Verification items for the finished model (mm, model axes). Face numbers are marked on the shaded views. A direction names the side the tool comes from. Give positions to 0.01 mm unless a question says otherwise; leave off trailing zeros. Write each loop counter-clockwise with the first axis right and the second up, starting at its lowest first coordinate (ties: lowest second). Pieces come first, ordered by that corner, then holes. Notation, with made-up numbers: M 13,3.5 L 69,3.5 A14 cw 69,24.5 Z; hole C 55.5,21.5 d6. An arc over 180 degrees is marked long. Answer as a JSON object with one key per item and string values.
```python
from build123d import *

# Parameters (mm, degrees)
SKETCH1_R           = 11.25
SKETCH1_R_2         = 1.6
BOSS_EXTRUDE1_DEPTH = 5
SKETCH4_R           = 2.8
CUT_EXTRUDE1_DEPTH  = 2.5
BOSS_EXTRUDE2_START = 11
SKETCH2_R           = 2.8
BOSS_EXTRUDE2_DEPTH = 11
BOSS_EXTRUDE3_DEPTH = 3
CHAMFER2_SIZE       = 1
CUT_EXTRUDE2_REACH  = 42.599
SKETCH5_R           = 2.1
SKETCH6_R           = 3.5
CUT_EXTRUDE3_DEPTH  = 7
CHAMFER3_SIZE       = 0.75


with BuildPart() as part:
    # Sketch1 → Boss-Extrude1 (new body)
    with BuildSketch(Plane(origin=(0, 0, 0), x_dir=(1, 0, 0), z_dir=(0, 1, 0))):
        Polygon((-20, 20.75), (-15, 20.75), (-14, 21.75), (-6, 21.75), (-5, 20.75), (5, 20.75), (6, 21.75), (14, 21.75), (15, 20.75), (20, 20.75), (20, -20.75), (-20, -20.75), align=None)
        with Locations(Location((0, 0, 0), (0, 0, 270))):
            Circle(SKETCH1_R, mode=Mode.SUBTRACT)
        with Locations(Location((15.5, 15.5, 0), (0, 0, 270))):
            Circle(SKETCH1_R_2, mode=Mode.SUBTRACT)
        with Locations(Location((-15.5, 15.5, 0), (0, 0, 270))):
            Circle(SKETCH1_R_2, mode=Mode.SUBTRACT)
        with Locations(Location((-15.5, -15.5, 0), (0, 0, 270))):
            Circle(SKETCH1_R_2, mode=Mode.SUBTRACT)
        with Locations(Location((15.5, -15.5, 0), (0, 0, 270))):
            Circle(SKETCH1_R_2, mode=Mode.SUBTRACT)
    extrude(amount=BOSS_EXTRUDE1_DEPTH)

    # Sketch4 → Cut-Extrude1 (cut)
    with BuildSketch(Plane(origin=(0, 5, 0), x_dir=(1, 0, 0), z_dir=(0, 1, 0))):
        with Locations(Location((-15.5, -15.5, 0), (0, 0, 270))):
            Circle(SKETCH4_R)
        with Locations(Location((15.5, 15.5, 0), (0, 0, 270))):
            Circle(SKETCH4_R)
        with Locations(Location((-15.5, 15.5, 0), (0, 0, 270))):
            Circle(SKETCH4_R)
        with Locations(Location((15.5, -15.5, 0), (0, 0, 270))):
            Circle(SKETCH4_R)
    extrude(amount=-CUT_EXTRUDE1_DEPTH, mode=Mode.SUBTRACT)

    # Sketch2 → Boss-Extrude2 (add)
    with BuildSketch(Plane(origin=(0, 5, 0), x_dir=(1, 0, 0), z_dir=(0, 1, 0)).offset(BOSS_EXTRUDE2_START)):
        with BuildLine():
            Line((-20, 10.75), (-8.968695557, 10.75))
            ThreePointArc((-8.968695557, 10.75), (0, 14), (8.968695557, 10.75))
            Line((8.968695557, 10.75), (20, 10.75))
            Line((20, 10.75), (20, 20.75))
            Line((20, 20.75), (15, 20.75))
            Line((15, 20.75), (14, 21.75))
            Line((14, 21.75), (6, 21.75))
            Line((6, 21.75), (5, 20.75))
            Line((5, 20.75), (-5, 20.75))
            Line((-5, 20.75), (-6, 21.75))
            Line((-6, 21.75), (-14, 21.75))
            Line((-14, 21.75), (-15, 20.75))
            Line((-15, 20.75), (-20, 20.75))
            Line((-20, 20.75), (-20, 10.75))
        make_face()
        with Locations((-15.5, 15.5)):
            Circle(SKETCH2_R, mode=Mode.SUBTRACT)
        with Locations((15.5, 15.5)):
            Circle(SKETCH2_R, mode=Mode.SUBTRACT)
    extrude(amount=-BOSS_EXTRUDE2_DEPTH)

    # Sketch3 → Boss-Extrude3 (add)
    with BuildSketch(Plane(origin=(20, 0, 0), x_dir=(0, 0, -1), z_dir=(1, 0, 0))):
        Polygon((10.75, 16), (-8.302558883, 5), (10.75, 5), align=None)
    boss_extrude3 = extrude(amount=-BOSS_EXTRUDE3_DEPTH)

    # Mirror1: Boss-Extrude3 across plane
    add(boss_extrude3.mirror(Plane(origin=(0, 0, 0), x_dir=(0, 0, 1), z_dir=(1, 0, 0))))

    # Chamfer2
    chamfer2_edges = [part.edges().sort_by_distance(p)[0] for p in [
        (12.984347779, 5, -10.75),
        (17, 5, -1.223720558),
        (-17, 5, -1.223720558),
        (0, 5, -14),
        (-12.984347779, 5, -10.75),
    ]]
    chamfer(chamfer2_edges, length=CHAMFER2_SIZE)

    # Sketch5 → Cut-Extrude2 (cut, up to next)
    with BuildSketch(Plane.XY.offset(-10.75), mode=Mode.PRIVATE) as cut_extrude2_sk1:
        with Locations((-10, 11)):
            Circle(SKETCH5_R)
    cut_extrude2_tool1 = extrude(cut_extrude2_sk1.sketch, amount=-CUT_EXTRUDE2_REACH, mode=Mode.PRIVATE) & part.part
    # Sketch5 → Cut-Extrude2 (cut, up to next)
    with BuildSketch(Plane.XY.offset(-10.75), mode=Mode.PRIVATE) as cut_extrude2_sk2:
        with Locations((10, 11)):
            Circle(SKETCH5_R)
    cut_extrude2_tool2 = extrude(cut_extrude2_sk2.sketch, amount=-CUT_EXTRUDE2_REACH, mode=Mode.PRIVATE) & part.part
    add(cut_extrude2_tool1.solids().sort_by_distance((-10, 11, -10.75))[0], mode=Mode.SUBTRACT)
    add(cut_extrude2_tool2.solids().sort_by_distance((10, 11, -10.75))[0], mode=Mode.SUBTRACT)

    # Sketch6 → Cut-Extrude3 (cut)
    with BuildSketch(Plane.XY.offset(-10.75)):
        with Locations((-10, 11)):
            Circle(SKETCH6_R)
        with Locations((10, 11)):
            Circle(SKETCH6_R)
    extrude(amount=-CUT_EXTRUDE3_DEPTH, mode=Mode.SUBTRACT)

    # Chamfer3
    chamfer3_edges = [part.edges().sort_by_distance(p)[0] for p in [
        (-17.5, 0, -20.75),
        (-14.5, 0, -21.25),
        (20, 5, 14.526279442),
        (-10, 0, -21.75),
        (20, 10.5, -1.223720558),
        (-5.5, 0, -21.25),
        (0, 0, -20.75),
        (-20, 5, 14.526279442),
        (-20, 10.5, -1.223720558),
        (5.5, 0, -21.25),
        (10, 0, -21.75),
        (14.5, 0, -21.25),
        (17.5, 0, -20.75),
        (20, 0, 0),
        (0, 0, 20.75),
        (-20, 0, 0),
        (20, 2.5, 20.75),
        (-20, 2.5, 20.75),
        (0, 0, -11.25),
        (15.5, 0, -17.1),
        (-15.5, 0, -17.1),
        (-15.5, 0, 13.9),
        (15.5, 0, 13.9),
        (0, 5, 20.75),
        (0, 16, -14),
        (20, 16, -15.75),
        (17.5, 16, -20.75),
        (14.5, 16, -21.25),
        (10, 16, -21.75),
        (5.5, 16, -21.25),
        (0, 16, -20.75),
        (-5.5, 16, -21.25),
        (-10, 16, -21.75),
        (-14.5, 16, -21.25),
        (-17.5, 16, -20.75),
        (-20, 16, -15.75),
    ]]
    chamfer(chamfer3_edges, length=CHAMFER3_SIZE)


solid = part.part
```
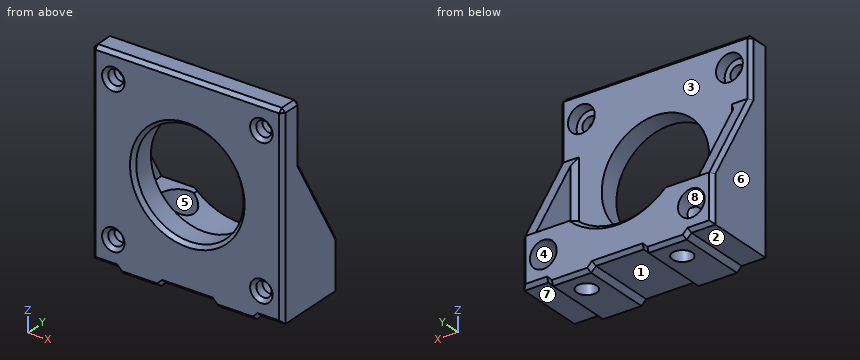
1) Access from +Z, -Z, +X, -X, +Y, -Y to the whole of each face (thin tool, end or side, straight path). Record for the marked faces 1, 2, 3, 4 and 5.
Completed:
{"face 1": "-Z, +Y, -Y", "face 2": "-Z, -X, +Y, -Y", "face 3": "+Z, +Y", "face 4": "+Y", "face 5": "+Z"}
2) Go/stop test with flat-tipped pins: pin 1 (1.5 mm diameter, centred on x = -18, y = 6, fed in from -Z); pin 2 (7.5 mm diameter, centred on x = -15.5, z = 15.5, fed in from +Y); pin 3 (2.5 mm diameter, centred on x = -11.5, y = 8.5, fed in from +Z). Record where each tip stops, or that it passes through.
Completed:
{"pin 1": "stops at z = -20.75", "pin 2": "stops at y = 5", "pin 3": "stops at z = -10.75"}
3) Section check B-B on y = 1.5. Record the boundary of the cut face in (x, z).
Completed:
{"outline": "M -20,-20.75 L -15,-20.75 L -14,-21.75 L -6,-21.75 L -5,-20.75 L 5,-20.75 L 6,-21.75 L 14,-21.75 L 15,-20.75 L 20,-20.75 L 20,20 L 19.25,20.75 L -19.25,20.75 L -20,20 Z; hole C -15.5,-15.5 d3.2; hole C -15.5,15.5 d3.2; hole C 0,0 d22.5; hole C 15.5,-15.5 d3.2; hole C 15.5,15.5 d3.2"}
4) Release check for a two-part mould opening along X. For the marked faces 6, 7 and 8 record: pulls with the +X half, pulls with the -X half, needs draft (parallel to the pull), parting line crosses it, or undercut.
Completed:
{"face 6": "pulls with the -X half", "face 7": "needs draft", "face 8": "undercut"}
5) Thickness scan on L1, parallel to Z at x = -15.5, y = 1.35; L2, parallel to X at y = 2.15, z = 15.5. Record the ranges inside material, lowest first.
Completed:
{"L1": "z = -20.75 to -17.1, -13.9 to 13.9, 17.1 to 20.75", "L2": "x = -20 to -17.1, -13.9 to 13.9, 17.1 to 20"}
6) Section check A-A on z = 15.5. Record the boundary of the cut face in (x, y), and give its area (3 significant figures).
Completed:
{"outline": "M -20,0.75 L -19.25,0 L -17.85,0 L -17.1,0.75 L -17.1,2.5 L -18.3,2.5 L -18.3,5 L -19.25,5 L -20,4.25 Z; M -13.9,0.75 L -13.15,0 L 13.15,0 L 13.9,0.75 L 13.9,2.5 L 12.7,2.5 L 12.7,5 L -12.7,5 L -12.7,2.5 L -13.9,2.5 Z; M 17.1,0.75 L 17.85,0 L 19.25,0 L 20,0.75 L 20,4.25 L 19.25,5 L 18.3,5 L 18.3,2.5 L 17.1,2.5 Z", "area": "154 mm2"}
7) Section check C-C on y = 11. Count the separate pieces of the cut face and the enclosed holes in it, and give its area (3 significant figures).
Completed:
{"separate pieces": "3", "enclosed holes": "0", "area": "257 mm2"}
